The listing builds one solid part. Answer for the finished solid, in the listing's coordinates (mm). Face numbers are marked on the shaded views. A direction names the side the tool comes from. Round coordinates to 2 decimals unless told otherwise and drop trailing zeros. Write each loop counter-clockwise with the first axis right and the second up, starting at its lowest first coordinate (ties: lowest second). Pieces come first, ordered by that corner, then holes. Notation, with made-up numbers: (18, -10.5) -> (31, -10.5) arc R22 ccw to (31, 7.5) -> close; hole circle Ø8 at (9.25, 83). An arc over 180 degrees is marked (long way). Write each question's results on one line, items separated by ' | '. Start each with the question number.
```python
from build123d import *

# Parameters (mm, degrees)
SKETCH1_W           = 80
SKETCH1_H           = 50
SKETCH1_R           = 1.65
BOSS_EXTRUDE1_DEPTH = 2
SKETCH2_W           = 55
SKETCH2_H           = 20
BOSS_EXTRUDE2_DEPTH = 10


with BuildPart() as part:
    # Sketch1 → Boss-Extrude1 (new body)
    with BuildSketch(Plane(origin=(0, 0, 0), x_dir=(1, 0, 0), z_dir=(0, 1, 0))):
        with Locations((40, 25)):
            Rectangle(SKETCH1_W, SKETCH1_H)
        with Locations(Location((2.625, 2.625, 0), (0, 0, 270))):
            Circle(SKETCH1_R, mode=Mode.SUBTRACT)
        with Locations(Location((77.375, 2.625, 0), (0, 0, 270))):
            Circle(SKETCH1_R, mode=Mode.SUBTRACT)
        with Locations(Location((2.625, 47.375, 0), (0, 0, 270))):
            Circle(SKETCH1_R, mode=Mode.SUBTRACT)
        with Locations(Location((77.375, 47.375, 0), (0, 0, 270))):
            Circle(SKETCH1_R, mode=Mode.SUBTRACT)
    extrude(amount=BOSS_EXTRUDE1_DEPTH)

    # Sketch2 → Boss-Extrude2 (add)
    with BuildSketch(Plane(origin=(0, 2, 0), x_dir=(1, 0, 0), z_dir=(0, 1, 0))):
        with Locations((40, 25)):
            Rectangle(SKETCH2_W, SKETCH2_H)
    extrude(amount=BOSS_EXTRUDE2_DEPTH)


solid = part.part
```
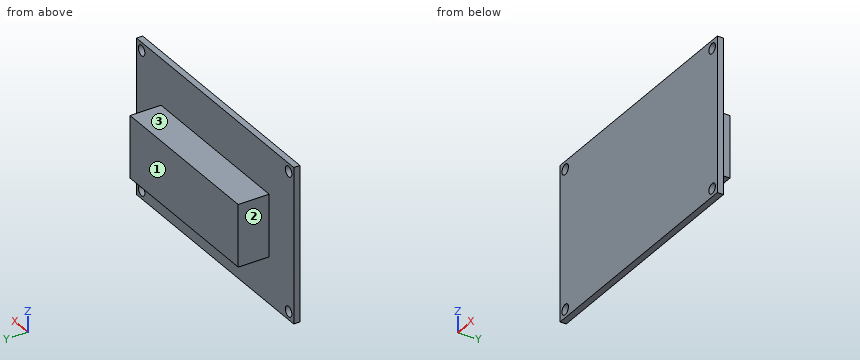
Q1. For the marked faces 1, 2 and 3, determine the directions among +Z, -Z, +X, -X, +Y, -Y from which every point of the face is accessible in a straight line to the end or side of a thin tool.
Q2. The part is cut by section A-A, the plane x = 49. Write down the section's boundary in (y, z).
Q3. The part is cut by section B-B, the plane z = -28.5. Write down the section's boundary in (x, y).
Q4. Find the intervals of material crossed by line 1 (X direction, y = 10.25, z = -33); line 2 (Y direction, x = 12, z = -43); line 3 (Z direction, x = 37, y = 11), in increasing order.
Q5. The part is cut by section D-D, the plane z = -41. Write down the section's boundary in (x, y).
Q6. Each of these flat-tipped pins is pushed along its axis until it touches: pin 1 (3 mm diameter, centred on y = 9, z = -21, fed in from +X); pin 2 (4 mm diameter, centred on x = 77.375, z = -2.625, fed in from +Y); pin 3 (3 mm diameter, centred on x = 46.5, y = 7.5, fed in from -Z). Where does it stop, or does it pass through?
Q7. The part is cut by section C-C, the plane y = 3.25. Write down the section's boundary in (x, z), then the cut area to 3 significant figures.
Answers follow:
1) face 1: +Z, -Z, +X, -X, +Y | face 2: +Z, -Z, -X, +Y | face 3: +Z, +X, -X, +Y
2) outline: (0, -50) -> (2, -50) -> (2, -35) -> (12, -35) -> (12, -15) -> (2, -15) -> (2, 0) -> (0, 0) -> close
3) outline: (0, 0) -> (80, 0) -> (80, 2) -> (67.5, 2) -> (67.5, 12) -> (12.5, 12) -> (12.5, 2) -> (0, 2) -> close
4) line 1: 12.5 to 67.5 | line 2: 0 to 2 | line 3: -35 to -15
5) outline: (0, 0) -> (80, 0) -> (80, 2) -> (0, 2) -> close
6) pin 1: x = 67.5 | pin 2: y = 2 | pin 3: z = -35
7) outline: (12.5, -35) -> (67.5, -35) -> (67.5, -15) -> (12.5, -15) -> close | area: 1,100 mm^2
